Design review of the part shown in the three views and the two pictorial views. Dimensions are in mm from the part's minimum x, y and z. A direction names the side the tool comes from. Round coordinates to 2 decimals unless told otherwise and drop trailing zeros. Loops run counter-clockwise (first coordinate to the right, second up) from the corner with the lowest first, then second, coordinate; pieces in that order, holes last. Notation, with made-up numbers: (-11.5, 7.5) - (22.5, 7.5) arc R35 ccw to (22.5, 40.5) - close; hole circle Ø10 at (-28, 48.25). An arc over 180 degrees is marked (long way). Return JSON: item names as keys, results as strings. Group by question number.
(1) Clearance check with flat-ended pins moving along their axes: pin 1 (1.8 mm diameter, centred on x = 11, y = 3, fed in from -Z); pin 2 (3.5 mm diameter, centred on x = 11, y = 19, fed in from +Z); pin 3 (6.5 mm diameter, centred on x = 11, y = 11, fed in from -Z); pin 4 (1.5 mm diameter, centred on y = 19, z = 0.5, fed in from -X). State where each tip first meets the part, or that it passes through.
(2) The part is to be moulded in two halves that separate along Y. For the marked faces 3, 4 and 5, say which applies: pulls with the +Y half, pulls with the -Y half, needs draft (parallel to the pull), parting line crosses it, or undercut.
(3) For the marked faces 1 and 2, list the 3-axis set-ups (+Z, -Z, +X, -X, +Y, -Y) from which the entire face can be reached by the end or side of a thin tool; tool diameter is ignored.
(4) We need section A-A, the plane y = 11. Write out the cut boundary in (x, z), and give its area (3 significant figures).
(5) We need section D-D, the plane y = 3. Write out the cut boundary in (x, z), and give its area (3 significant figures).
(6) We need section C-C, the plane z = 1.25. Write out the cut boundary in (x, y).
(7) Wall thickness on L1, parallel to Y at x = 11, z = 1.15; L2, parallel to X at y = 11.25, z = 3.05; L3, parallel to Z at x = 17.5, y = 5.75: over which ranges is each line inside the solid? List them lowest first. Write a range as [from, to].
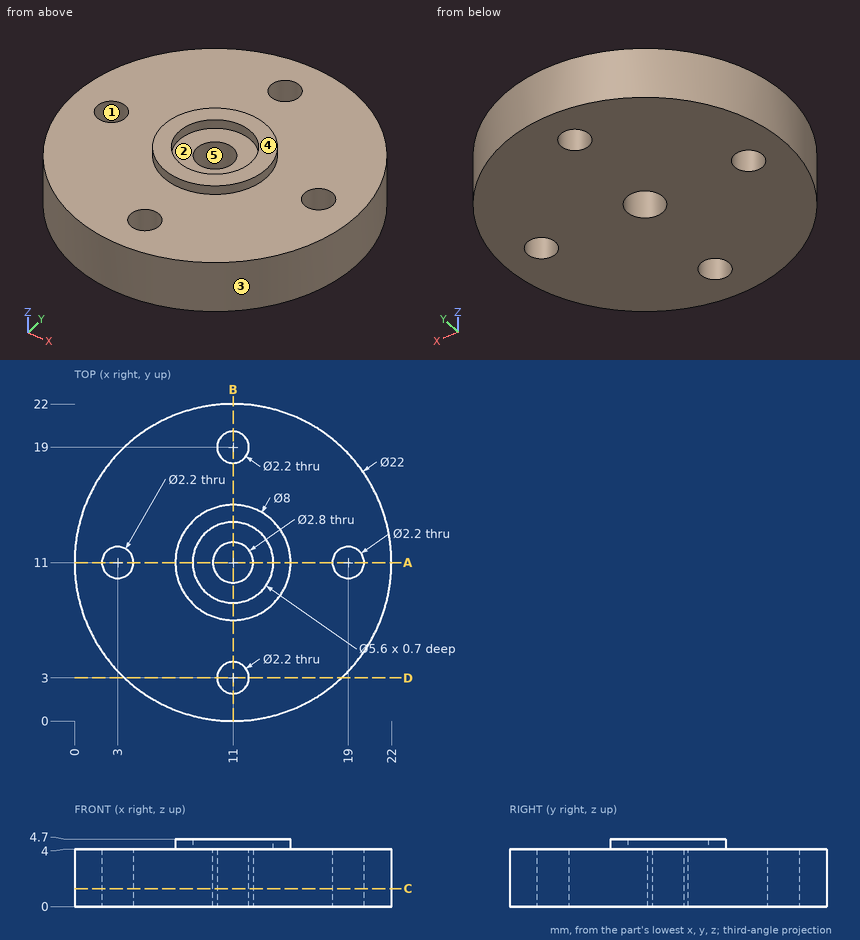
Solutions:
{
 "1": {"pin 1": "through", "pin 2": "z = 4", "pin 3": "z = 0", "pin 4": "x = 2.73"},
 "2": {"face 3": "parting line crosses it", "face 4": "needs draft", "face 5": "undercut"},
 "3": {"face 1": "+Z, -Z", "face 2": "+Z"},
 "4": {"outline": "(0, 0) - (1.9, 0) - (1.9, 4) - (0, 4) - close; (4.1, 0) - (9.6, 0) - (9.6, 4) - (8.2, 4) - (8.2, 4.7) - (7, 4.7) - (7, 4) - (4.1, 4) - close; (12.4, 0) - (17.9, 0) - (17.9, 4) - (15, 4) - (15, 4.7) - (13.8, 4.7) - (13.8, 4) - (12.4, 4) - close; (20.1, 0) - (22, 0) - (22, 4) - (20.1, 4) - close", "area": "60.9 mm^2"},
 "5": {"outline": "(3.45, 0) - (9.9, 0) - (9.9, 4) - (3.45, 4) - close; (12.1, 0) - (18.55, 0) - (18.55, 4) - (12.1, 4) - close", "area": "51.6 mm^2"},
 "6": {"outline": "circle Ø22 at (11, 11); hole circle Ø2.2 at (3, 11); hole circle Ø2.8 at (11, 11); hole circle Ø2.2 at (11, 3); hole circle Ø2.2 at (11, 19); hole circle Ø2.2 at (19, 11)"},
 "7": {"L1": "[0, 1.9], [4.1, 9.6], [12.4, 17.9], [20.1, 22]", "L2": "[0, 1.93], [4.07, 9.62], [12.38, 17.93], [20.07, 22]", "L3": "[0, 4]"}
}
